from build123d import *

# Parameters (mm, degrees)
BOSS_EXTRUDE1_DEPTH = 3.175
SKETCH2_R           = 3.175
SKETCH2_R_2         = 6.35
SKETCH2_R_3         = 13
SKETCH2_R_4         = 1.5875
SKETCH2_R_5         = 2.032
CUT_EXTRUDE1_DEPTH  = 4.175
FILLET1_R           = 25.4


with BuildPart() as part:
    # Sketch1 → Boss-Extrude1 (new body)
    with BuildSketch(Plane(origin=(0, 0, 0), x_dir=(0, 0, -1), z_dir=(1, 0, 0))):
        with BuildLine():
            Line((-85.725, -120.65), (-111.65780492, -113.349682952))
            ThreePointArc((-111.65780492, -113.349682952), (-130.175, -88.9), (-111.65780492, -64.450317048))
            Line((-111.65780492, -64.450317048), (-85.725, -57.15))
            Line((-85.725, -57.15), (-85.725, 120.65))
            Line((-85.725, 120.65), (85.725, 120.65))
            Line((85.725, 120.65), (85.725, -120.65))
            Line((85.725, -120.65), (-85.725, -120.65))
        make_face()
    extrude(amount=BOSS_EXTRUDE1_DEPTH)

    # Sketch2 → Cut-Extrude1 (cut, through all)
    with BuildSketch(Plane(origin=(3.175, 0, 0), x_dir=(0, 0, -1), z_dir=(1, 0, 0))):
        with Locations((73.025, -107.95)):
            Circle(SKETCH2_R)
        with Locations((73.025, -35.983333333)):
            Circle(SKETCH2_R)
        with Locations((73.025, 35.983333333)):
            Circle(SKETCH2_R)
        with Locations((73.025, 107.95)):
            Circle(SKETCH2_R)
        with Locations((-55.88, -101.6)):
            Circle(SKETCH2_R_2)
        with Locations((-55.88, -50.8)):
            Circle(SKETCH2_R_2)
        with Locations((-55.88, 0)):
            Circle(SKETCH2_R_2)
        with Locations((-55.88, 50.8)):
            Circle(SKETCH2_R_2)
        with Locations((-55.88, 101.6)):
            Circle(SKETCH2_R_2)
        with Locations((-36.83, -76.2)):
            Circle(SKETCH2_R)
        with Locations((-36.83, -25.4)):
            Circle(SKETCH2_R)
        with Locations((-36.83, 25.4)):
            Circle(SKETCH2_R)
        with Locations((-36.83, 76.2)):
            Circle(SKETCH2_R)
        with Locations((-104.775, -88.9)):
            Circle(SKETCH2_R_3)
        with Locations((-104.775, -73.4)):
            Circle(SKETCH2_R_4)
        with Locations((-97.025, -75.476606241)):
            Circle(SKETCH2_R_4)
        with Locations((-91.351606241, -81.15)):
            Circle(SKETCH2_R_4)
        with Locations((-89.275, -88.9)):
            Circle(SKETCH2_R_4)
        with Locations((-91.351606241, -96.65)):
            Circle(SKETCH2_R_4)
        with Locations((-97.025, -102.323393759)):
            Circle(SKETCH2_R_4)
        with Locations((-104.775, -104.4)):
            Circle(SKETCH2_R_4)
        with Locations((-112.525, -102.323393759)):
            Circle(SKETCH2_R_4)
        with Locations((-118.198393759, -96.65)):
            Circle(SKETCH2_R_4)
        with Locations((-120.275, -88.9)):
            Circle(SKETCH2_R_4)
        with Locations((-118.198393759, -81.15)):
            Circle(SKETCH2_R_4)
        with Locations((-112.525, -75.476606241)):
            Circle(SKETCH2_R_4)
        with Locations((6.35, 103.1875)):
            Circle(SKETCH2_R_5)
        with Locations((50.8, 103.1875)):
            Circle(SKETCH2_R_5)
        with Locations((50.8, -100.0125)):
            Circle(SKETCH2_R_4)
        with Locations((6.35, -100.0125)):
            Circle(SKETCH2_R_4)
    extrude(amount=-CUT_EXTRUDE1_DEPTH, mode=Mode.SUBTRACT)

    # Fillet1
    fillet1_edges = [part.edges().sort_by_distance(p)[0] for p in [
        (1.5875, -120.65, 85.725),
        (1.5875, -57.15, 85.725),
        (1.5875, 120.65, 85.725),
    ]]
    fillet(fillet1_edges, radius=FILLET1_R)


solid = part.part
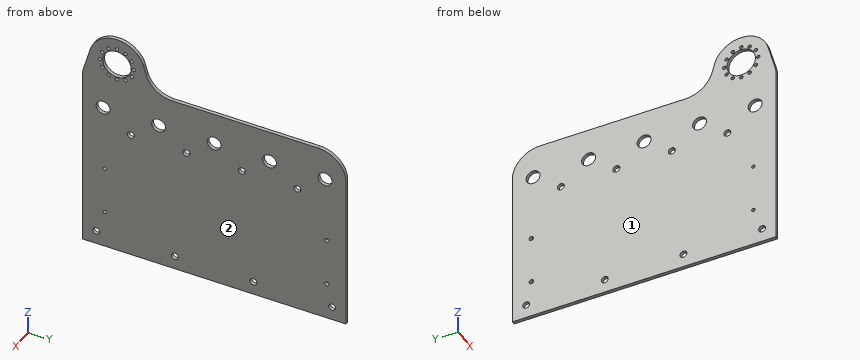
For this review, take the finished solid that the model builds, in its own axes (mm). Face numbers are marked on the shaded views. Give positions to 0.01 mm unless a question says otherwise; leave off trailing zeros. Loops run counter-clockwise (first coordinate to the right, second up) from the corner with the lowest first, then second, coordinate; pieces in that order, holes last.
Item 1: Draft analysis for pull direction X (two halves, no side actions). For the marked faces 1 and 2, state which applies: +X half, -X half, draft (parallel to the pull), parting line (faces both ways), or undercut.
Item 2: Take a section at B-B, the plane y = 50.8. State the section outline as (x, z) points (3 decimals), and give its area (3 significant figures).
Item 3: Take a section at D-D, the plane x = 0.8. Give the number of separate pieces and of enclosed holes in the cut face, and give its area (3 significant figures).
Item 4: For line 1 along Y through (x, z) = (2.4, 55.88); line 2 along Y through (x, z) = (1.35, -50.5); line 3 along Z through (x, y) = (1.3, -16.5) (3 decimals), list the stretches that pass through material, from the lowest coordinate up.
Item 5: Insertion check: pin 1 (4 mm diameter, centred on y = -65, z = 84.5, fed in from -X); pin 2 (1.5 mm diameter, centred on x = 2, y = 67.5, fed in from +Z) (3 decimals). Each pin has a flat end and moves straight along its axis. Give the tip position at first contact, or say it passes through.
Item 6: Take a section at A-A, the plane z = 36.83. State the section outline as (x, y) points (3 decimals).
Item 7: Take a section at C-C, the plane y = 25.4. State the section outline as (x, z) points (3 decimals).
Calculated:
1. face 1: -X half
1. face 2: +X half
2. outline: (0, -85.725) - (3.175, -85.725) - (3.175, 49.53) - (0, 49.53) - close; (0, 62.23) - (3.175, 62.23) - (3.175, 85.725) - (0, 85.725) - close
2. area: 504 mm2
3. separate pieces: 1
3. enclosed holes: 30
3. area: 41,900 mm2
4. line 1: y = -120.65 to -107.95, -95.25 to -57.15, -44.45 to -6.35, 6.35 to 44.45, 57.15 to 95.25, 107.95 to 120.65
4. line 2: y = -120.65 to -101.57, -98.45 to 101.18, 105.2 to 120.65
4. line 3: z = -85.725 to 85.725
5. pin 1: stops at x = 0
5. pin 2: stops at z = 85.725
6. outline: (0, -120.65) - (3.175, -120.65) - (3.175, -79.375) - (0, -79.375) - close; (0, -73.025) - (3.175, -73.025) - (3.175, -28.575) - (0, -28.575) - close; (0, -22.225) - (3.175, -22.225) - (3.175, 22.225) - (0, 22.225) - close; (0, 28.575) - (3.175, 28.575) - (3.175, 73.025) - (0, 73.025) - close; (0, 79.375) - (3.175, 79.375) - (3.175, 120.65) - (0, 120.65) - close
7. outline: (0, -85.725) - (3.175, -85.725) - (3.175, 33.655) - (0, 33.655) - close; (0, 40.005) - (3.175, 40.005) - (3.175, 85.725) - (0, 85.725) - close
